from build123d import *

# Parameters (mm, degrees)
ESQUISSE1_R        = 1.5
ESQUISSE1_R_2      = 4
ESQUISSE1_R_3      = 3
BOSS_EXTRU_1_DEPTH = 3
ESQUISSE2_R        = 5
ESQUISSE2_R_2      = 4
BOSS_EXTRU_2_DEPTH = 10


with BuildPart() as part:
    # Esquisse1 → Boss.-Extru.1 (new body)
    with BuildSketch(Plane(origin=(0, 0, 0), x_dir=(1, 0, 0), z_dir=(0, 1, 0))):
        with BuildLine():
            Line((-4, 4.472135955), (-4, -4.472135955))
            ThreePointArc((-4, -4.472135955), (0, -6), (4, -4.472135955))
            Line((4, -4.472135955), (4, 4.472135955))
            Line((4, 4.472135955), (4, 40.527864045))
            ThreePointArc((4, 40.527864045), (5.543277195, 47.296100594), (-0.333850535, 50.990704785))
            Line((-0.333850535, 50.990704785), (-3.201683371, 53.85853762))
            ThreePointArc((-3.201683371, 53.85853762), (-13.435028843, 58.435028843), (-8.85853762, 48.201683371))
            Line((-8.85853762, 48.201683371), (-5.990704785, 45.333850535))
            ThreePointArc((-5.990704785, 45.333850535), (-5.543277195, 42.703899406), (-4, 40.527864045))
            Line((-4, 40.527864045), (-4, 4.472135955))
        make_face()
        with Locations(Location((0, 0, 0), (0, 0, 270))):
            Circle(ESQUISSE1_R, mode=Mode.SUBTRACT)
        with Locations((-9.192388155, 54.192388155)):
            Circle(ESQUISSE1_R_2, mode=Mode.SUBTRACT)
        with Locations(Location((0, 45, 0), (0, 0, 270))):
            Circle(ESQUISSE1_R, mode=Mode.SUBTRACT)
        with Locations((-9.192388155, 54.192388155)):
            Circle(ESQUISSE1_R_2)
        with Locations(Location((-9.192388155, 54.192388155, 0), (0, 0, 270))):
            Circle(ESQUISSE1_R_3, mode=Mode.SUBTRACT)
    extrude(amount=BOSS_EXTRU_1_DEPTH)

    # Esquisse2 → Boss.-Extru.2 (add)
    with BuildSketch(Plane(origin=(0, 3, 0), x_dir=(1, 0, 0), z_dir=(0, 1, 0))):
        with Locations(Location((-9.192388155, 54.192388155, 0), (0, 0, 270))):
            Circle(ESQUISSE2_R)
        with Locations(Location((-9.192388155, 54.192388155, 0), (0, 0, 270))):
            Circle(ESQUISSE2_R_2, mode=Mode.SUBTRACT)
    extrude(amount=BOSS_EXTRU_2_DEPTH)


solid = part.part
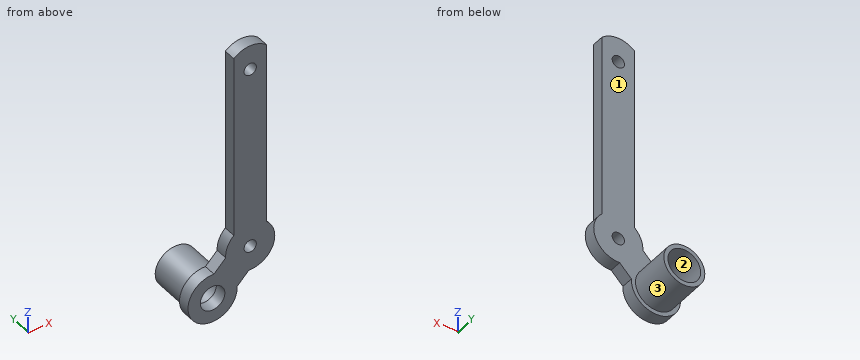
Geometry: final body of the model. Coordinates: model frame, mm. Face numbers are marked on the shaded views. Coordinates: 2 decimals unless noted, no trailing zeros. Loops run counter-clockwise (first coordinate to the right, second up) from the corner with the lowest first, then second, coordinate; pieces in that order, holes last. Notation, with made-up numbers: M 74,67 L 91,67 A16 cw 91,80 Z; hole C 49.25,-34.5 d8. An arc over 180 degrees is marked long. One line per item, written item: value. Start each with the question number.
1) Cut plane D-D (x = 3.25). Return loops of the section in (y, z).
2) Cut plane C-C (z = -56). Return loops of the section in (x, y), then the cut area to 3 significant figures.
3) Pin query (flat end, axial travel): P1, Ø1, axis at x = -6, z = -45.5, coming from the +Y side; P2, Ø2.5, axis at y = 2, z = -16.5, coming from the +X side; P3, Ø3.5, axis at y = 1.5, z = -8, coming from the -X side. Return the tip coordinate at first contact, or that it passes through.
4) Draft query along Z for the marked faces 1, 2 and 3. Return one class per face: released by +Z, released by -Z, zero draft, split by the parting line, or undercut.
5) Cut plane A-A (z = 0). Return loops of the section in (x, y), then the cut area to 3 significant figures.
6) Cut plane B-B (y = 7). Return loops of the section in (x, z).
7) Material intervals for L1, parallel to X at y = 2.3, z = -45; L2, parallel to X at y = 1.95, z = 0; L3, parallel to X at y = 2, z = -2, sorted ascending. Write a range as from..to.
Evaluation:
1. outline: M 0,-50.04 L 3,-50.04 L 3,5.04 L 0,5.04 Z
2. outline: M -14.91,0 L -11.59,0 L -11.59,3 L -12.76,3 L -12.76,13 L -13.85,13 L -13.85,3 L -14.91,3 Z; M -6.8,0 L -3.47,0 L -3.47,3 L -4.53,3 L -4.53,13 L -5.62,13 L -5.62,3 L -6.8,3 Z
2. area: 41.8 mm^2
3. P1: y = 3
3. P2: x = 4
3. P3: x = -4
4. face 1: zero draft
4. face 2: undercut
4. face 3: split by the parting line
5. outline: M -4,0 L -1.5,0 L -1.5,3 L -4,3 Z; M 1.5,0 L 4,0 L 4,3 L 1.5,3 Z
5. area: 15.0 mm^2
6. outline: C -9.19,-54.19 d10; hole C -9.19,-54.19 d8
7. L1: -6..-1.5, 1.5..6
7. L2: -4..-1.5, 1.5..4
7. L3: -4..4
